Build history of the part. All positions in model axes, mm. Face numbers are marked on the shaded views. Give positions to 0.01 mm unless a question says otherwise; leave off trailing zeros. Order: outer loops, then holes, each group sorted by start corner. A loop starts at its lowest first (then second) coordinate and runs counter-clockwise, first axis right, second up. Notation, with made-up numbers: (46.5, 53.25) - (93.5, 53.25) arc R22 ccw to (93.5, 79.25) - close; hole circle Ø10 at (2, 4). An arc over 180 degrees is marked (long way). Answer in a Markdown table with one row per item.
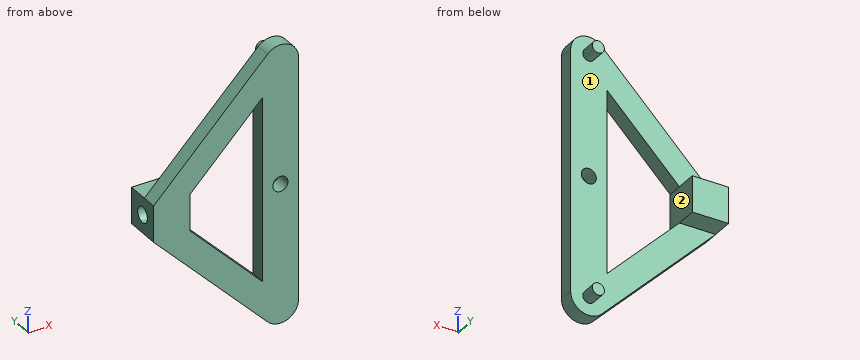
```python
from build123d import *

# Parameters (mm, degrees)
BOSS_EXTRUDE4_DEPTH = 3.175
SKETCH11_W          = 7.62
SKETCH11_H          = 7.62
BOSS_EXTRUDE5_DEPTH = 7.62
SKETCH13_R          = 1.27
BOSS_EXTRUDE6_DEPTH = 3.302
CUT_EXTRUDE3_REACH  = 41.803
SKETCH14_R          = 1.5875
SKETCH16_R          = 1.651
CUT_EXTRUDE4_DEPTH  = 3.81


with BuildPart() as part:
    # Sketch10 → Boss-Extrude4 (new body)
    with BuildSketch(Plane(origin=(0, 0, 0), x_dir=(1, 0, 0), z_dir=(0, 1, 0))):
        with BuildLine():
            Line((-3.81, 19.245944402), (-3.81, -19.245944402))
            Line((-3.81, -19.245944402), (-19.05, -3.81))
            Line((-19.05, -3.81), (-26.67, -3.81))
            Line((-26.67, -3.81), (-2.711230101, -28.076813654))
            ThreePointArc((-2.711230101, -28.076813654), (1.44677457, -28.924619603), (3.81, -25.4))
            Line((3.81, -25.4), (3.81, 25.4))
            ThreePointArc((3.81, 25.4), (1.44677457, 28.924619603), (-2.711230101, 28.076813654))
            Line((-2.711230101, 28.076813654), (-26.67, 3.81))
            Line((-26.67, 3.81), (-19.05, 3.81))
            Line((-19.05, 3.81), (-3.81, 19.245944402))
        make_face()
    extrude(amount=BOSS_EXTRUDE4_DEPTH)

    # Sketch11 → Boss-Extrude5 (add)
    with BuildSketch(Plane(origin=(0, 0, 0), x_dir=(1, 0, 0), z_dir=(0, 1, 0))):
        with Locations((-22.86, 0)):
            Rectangle(SKETCH11_W, SKETCH11_H)
    extrude(amount=BOSS_EXTRUDE5_DEPTH)

    # Sketch13 → Boss-Extrude6 (add)
    with BuildSketch(Plane(origin=(0, 3.175, 0), x_dir=(1, 0, 0), z_dir=(0, 1, 0))):
        with Locations(Location((0, -25.4, 0), (0, 0, 90))):
            Circle(SKETCH13_R)
        with Locations(Location((0, 25.4, 0), (0, 0, 90))):
            Circle(SKETCH13_R)
    extrude(amount=BOSS_EXTRUDE6_DEPTH)

    # Sketch14 → Cut-Extrude3 (cut, up to next)
    with BuildSketch(Plane(origin=(0, 3.175, 0), x_dir=(1, 0, 0), z_dir=(0, 1, 0)), mode=Mode.PRIVATE) as cut_extrude3_sk1:
        with Locations(Location((0, 0, 0), (0, 0, 270))):
            Circle(SKETCH14_R)
    cut_extrude3_tool1 = extrude(cut_extrude3_sk1.sketch, amount=-CUT_EXTRUDE3_REACH, mode=Mode.PRIVATE) & part.part
    add(cut_extrude3_tool1.solids().sort_by_distance((0, 3.175, 0))[0], mode=Mode.SUBTRACT)

    # Sketch16 → Cut-Extrude4 (cut)
    with BuildSketch(Plane.ZY.offset(26.67)):
        with Locations((0, 3.81)):
            Circle(SKETCH16_R)
    extrude(amount=-CUT_EXTRUDE4_DEPTH, mode=Mode.SUBTRACT)


solid = part.part
```
1. Cut at A-A on x = 0. Write the cut outline in (y, z) (1 decimal), and give its area (3 significant figures).
Check result:
| item | result |
|---|---|
| outline | (0, -29.2) - (3.2, -29.2) - (3.2, -26.7) - (6.5, -26.7) - (6.5, -24.1) - (3.2, -24.1) - (3.2, -1.6) - (0, -1.6) - close; (0, 1.6) - (3.2, 1.6) - (3.2, 24.1) - (6.5, 24.1) - (6.5, 26.7) - (3.2, 26.7) - (3.2, 29.2) - (0, 29.2) - close |
| area | 192 mm² |
2. Cut at D-D on z = -12. Write the cut outline in (x, y) (3 decimals), and give its area (3 significant figures).
Check result:
| item | result |
|---|---|
| outline | (-18.584, 0) - (-10.964, 0) - (-10.964, 3.175) - (-18.584, 3.175) - close; (-3.81, 0) - (3.81, 0) - (3.81, 3.175) - (-3.81, 3.175) - close |
| area | 48.4 mm² |
3. Cut at C-C on y = 3.81. Write the cut outline in (x, z), and give its area (3 significant figures).
Check result:
| item | result |
|---|---|
| outline | (-26.67, -3.81) - (-19.05, -3.81) - (-19.05, 3.81) - (-26.67, 3.81) - (-26.67, 1.65) - (-22.86, 1.65) - (-22.86, -1.65) - (-26.67, -1.65) - close; circle Ø2.54 at (0, -25.4); circle Ø2.54 at (0, 25.4) |
| area | 55.6 mm² |
4. Probe line 1 (X direction, y = 1.6, z = 0); line 2 (Y direction, x = -8.5, z = -21) (3 decimals); line 3 (Z direction, x = -7.5, y = 2.75). List the from-to ranges inside material, lowest first.
Check result:
| item | result |
|---|---|
| line 1 | x = -26.67 to -19.05, -3.81 to -1.59, 1.59 to 3.81 |
| line 2 | y = 0 to 3.175 |
| line 3 | z = -23.23 to -15.51, 15.51 to 23.23 |
5. Two-plate mould, pull along X, no slides. Class the marked faces 1 and 2: +X half, -X half, draft (parallel to the pull), parting line (faces both ways), or undercut.
Check result:
| item | result |
|---|---|
| face 1 | draft |
| face 2 | undercut |
6. Drop flat-ended pins along their axis: P1, Ø9, axis at x = -8.5, z = -12.5, coming from the +Y side (3 decimals); P2, Ø2.5, axis at y = 1, z = 4.5, coming from the -X side; P3, Ø2, axis at x = -4.5, y = 4, coming from the -Z side; P4, Ø3, axis at x = -11.5, y = 2.5, coming from the -Z side. Give the stop position or say it passes through.
Check result:
| item | result |
|---|---|
| P1 | stops at y = 3.175 |
| P2 | stops at x = -26.67 |
| P3 | stops at z = -26.84 |
| P4 | stops at z = -20.69 |
7. Cut at B-B on z = 0. Count the separate pieces of the cut face and the enclosed holes in it, and give its area (3 significant figures).
Check result:
| item | result |
|---|---|
| separate pieces | 3 |
| enclosed holes | 0 |
| area | 59.6 mm² |
